```python
from build123d import *

# Parameters (mm, degrees)
BOSS_EXTRUDE1_DEPTH       = 6.35
F_6_CLEARANCE_HOLE1_D     = 3.6576
F_6_CLEARANCE_HOLE1_DEPTH = 25.4
F_6_CLEARANCE_HOLE1_TIP   = 1.0988539
FILLET1_R                 = 12.7
F_4_CLEARANCE_HOLE1_D     = 2.9464
F_4_CLEARANCE_HOLE1_DEPTH = 25.4
F_4_CLEARANCE_HOLE1_TIP   = 0.885187864
LPATTERN4_COUNT           = 6
LPATTERN4_PITCH           = 25.4
LPATTERN4_COUNT_DIR2      = 7
LPATTERN4_PITCH_DIR2      = 23.622


with BuildPart() as part:
    # Sketch1 → Boss-Extrude1 (new body)
    with BuildSketch(Plane(origin=(0, 0, 0), x_dir=(1, 0, 0), z_dir=(0, 1, 0))):
        with BuildLine():
            Line((65.058096917, 37.174573643), (142.24566953, 81.28))
            ThreePointArc((142.24566953, 81.28), (0, 163.83), (-142.24566953, 81.28))
            Line((-142.24566953, 81.28), (-65.058096917, 37.174573643))
            ThreePointArc((-65.058096917, 37.174573643), (0, 74.93), (65.058096917, 37.174573643))
        make_face()
    extrude(amount=BOSS_EXTRUDE1_DEPTH)

    # 6 Clearance Hole1
    with Locations(Plane(origin=(-50.8, 6.35, -125.73), x_dir=(0, 0, 1), z_dir=(0, 1, 0))):
        with Locations((0, 0), (0, 101.6)):
            Hole(F_6_CLEARANCE_HOLE1_D / 2, depth=F_6_CLEARANCE_HOLE1_DEPTH)
            with Locations((0, 0, -(F_6_CLEARANCE_HOLE1_DEPTH + F_6_CLEARANCE_HOLE1_TIP / 2))):  # 118° drill point
                Cone(0, F_6_CLEARANCE_HOLE1_D / 2, F_6_CLEARANCE_HOLE1_TIP, mode=Mode.SUBTRACT)

    # Fillet1
    fillet1_edges = [part.edges().sort_by_distance(p)[0] for p in [
        (142.24566953, 3.175, -81.28),
        (65.058096917, 3.175, -37.174573643),
        (-65.058096917, 3.175, -37.174573643),
        (-142.24566953, 3.175, -81.28),
    ]]
    fillet(fillet1_edges, radius=FILLET1_R)

    # 4 Clearance Hole1
    with Locations(Plane(origin=(0, 6.35, 0), x_dir=(-1, 0, 0), z_dir=(0, 1, 0))):
        with Locations((-34.0106, -133.35), (34.0106, -133.35)):
            Hole(F_4_CLEARANCE_HOLE1_D / 2, depth=F_4_CLEARANCE_HOLE1_DEPTH)
            with Locations((0, 0, -(F_4_CLEARANCE_HOLE1_DEPTH + F_4_CLEARANCE_HOLE1_TIP / 2))):  # 118° drill point
                Cone(0, F_4_CLEARANCE_HOLE1_D / 2, F_4_CLEARANCE_HOLE1_TIP, mode=Mode.SUBTRACT)

    # Sketch5 → 10 Clearance Hole1 (revolve, cut)
    with BuildSketch(Plane(origin=(-128.255094273, 6.35, -84.874017323), x_dir=(0, 0, 1), z_dir=(1, 0, 0))):
        Polygon((0, 0), (0, 26.895662253), (2.4892, 25.4), (2.4892, 0), align=None)
    f_10_clearance_hole1 = revolve(axis=Axis((-128.255094273, 12.7, -84.874017323), (0, -1, 0)), mode=Mode.SUBTRACT)

    # LPattern4: 10 Clearance Hole1 6 × 7, 28 skipped
    with Locations(*[Vector(0, 0, -1) * (i * LPATTERN4_PITCH) + Vector(0.8667949394357126, 0, 0.49866475007628064) * (j * LPATTERN4_PITCH_DIR2) for i in range(LPATTERN4_COUNT) for j in range(LPATTERN4_COUNT_DIR2) if (i, j) not in ((0, 0), (0, 4), (0, 5), (0, 6), (1, 0), (1, 4), (1, 5), (1, 6), (2, 0), (2, 1), (2, 4), (2, 6), (3, 0), (3, 1), (3, 2), (3, 4), (3, 6), (4, 0), (4, 1), (4, 2), (4, 3), (4, 4), (4, 6), (5, 0), (5, 1), (5, 2), (5, 3), (5, 4), (5, 6))]):
        add(f_10_clearance_hole1, mode=Mode.SUBTRACT)

    # Mirror4: 10 Clearance Hole1 across plane
    add(f_10_clearance_hole1.mirror(Plane(origin=(0, 0, 0), x_dir=(0, 0, 1), z_dir=(1, 0, 0))), mode=Mode.SUBTRACT)

    # Mirror4 copy 1 sketch → Mirror4 copy 1 (revolve, cut)
    with BuildSketch(Plane(origin=(107.779664214, 6.35, -73.094558596), x_dir=(0, 0, 1), z_dir=(-1, 0, 0))):
        Polygon((0, 0), (0, -26.895662253), (2.4892, -25.4), (2.4892, 0), align=None)
    revolve(axis=Axis((107.779664214, 12.7, -73.094558596), (0, 1, 0)), mode=Mode.SUBTRACT)

    # Mirror4 copy 2 sketch → Mirror4 copy 2 (revolve, cut)
    with BuildSketch(Plane(origin=(87.304234155, 6.35, -61.31509987), x_dir=(0, 0, 1), z_dir=(-1, 0, 0))):
        Polygon((0, 0), (0, -26.895662253), (2.4892, -25.4), (2.4892, 0), align=None)
    revolve(axis=Axis((87.304234155, 12.7, -61.31509987), (0, 1, 0)), mode=Mode.SUBTRACT)

    # Mirror4 copy 3 sketch → Mirror4 copy 3 (revolve, cut)
    with BuildSketch(Plane(origin=(66.828804095, 6.35, -49.535641144), x_dir=(0, 0, 1), z_dir=(-1, 0, 0))):
        Polygon((0, 0), (0, -26.895662253), (2.4892, -25.4), (2.4892, 0), align=None)
    revolve(axis=Axis((66.828804095, 12.7, -49.535641144), (0, 1, 0)), mode=Mode.SUBTRACT)

    # Mirror4 copy 4 sketch → Mirror4 copy 4 (revolve, cut)
    with BuildSketch(Plane(origin=(107.779664214, 6.35, -98.494558596), x_dir=(0, 0, 1), z_dir=(-1, 0, 0))):
        Polygon((0, 0), (0, -26.895662253), (2.4892, -25.4), (2.4892, 0), align=None)
    revolve(axis=Axis((107.779664214, 12.7, -98.494558596), (0, 1, 0)), mode=Mode.SUBTRACT)

    # Mirror4 copy 5 sketch → Mirror4 copy 5 (revolve, cut)
    with BuildSketch(Plane(origin=(87.304234155, 6.35, -86.71509987), x_dir=(0, 0, 1), z_dir=(-1, 0, 0))):
        Polygon((0, 0), (0, -26.895662253), (2.4892, -25.4), (2.4892, 0), align=None)
    revolve(axis=Axis((87.304234155, 12.7, -86.71509987), (0, 1, 0)), mode=Mode.SUBTRACT)

    # Mirror4 copy 6 sketch → Mirror4 copy 6 (revolve, cut)
    with BuildSketch(Plane(origin=(66.828804095, 6.35, -74.935641144), x_dir=(0, 0, 1), z_dir=(-1, 0, 0))):
        Polygon((0, 0), (0, -26.895662253), (2.4892, -25.4), (2.4892, 0), align=None)
    revolve(axis=Axis((66.828804095, 12.7, -74.935641144), (0, 1, 0)), mode=Mode.SUBTRACT)

    # Mirror4 copy 7 sketch → Mirror4 copy 7 (revolve, cut)
    with BuildSketch(Plane(origin=(87.304234155, 6.35, -112.11509987), x_dir=(0, 0, 1), z_dir=(-1, 0, 0))):
        Polygon((0, 0), (0, -26.895662253), (2.4892, -25.4), (2.4892, 0), align=None)
    revolve(axis=Axis((87.304234155, 12.7, -112.11509987), (0, 1, 0)), mode=Mode.SUBTRACT)

    # Mirror4 copy 8 sketch → Mirror4 copy 8 (revolve, cut)
    with BuildSketch(Plane(origin=(66.828804095, 6.35, -100.335641144), x_dir=(0, 0, 1), z_dir=(-1, 0, 0))):
        Polygon((0, 0), (0, -26.895662253), (2.4892, -25.4), (2.4892, 0), align=None)
    revolve(axis=Axis((66.828804095, 12.7, -100.335641144), (0, 1, 0)), mode=Mode.SUBTRACT)

    # Mirror4 copy 9 sketch → Mirror4 copy 9 (revolve, cut)
    with BuildSketch(Plane(origin=(25.877943977, 6.35, -76.776723691), x_dir=(0, 0, 1), z_dir=(-1, 0, 0))):
        Polygon((0, 0), (0, -26.895662253), (2.4892, -25.4), (2.4892, 0), align=None)
    revolve(axis=Axis((25.877943977, 12.7, -76.776723691), (0, 1, 0)), mode=Mode.SUBTRACT)

    # Mirror4 copy 10 sketch → Mirror4 copy 10 (revolve, cut)
    with BuildSketch(Plane(origin=(66.828804095, 6.35, -125.735641144), x_dir=(0, 0, 1), z_dir=(-1, 0, 0))):
        Polygon((0, 0), (0, -26.895662253), (2.4892, -25.4), (2.4892, 0), align=None)
    revolve(axis=Axis((66.828804095, 12.7, -125.735641144), (0, 1, 0)), mode=Mode.SUBTRACT)

    # Mirror4 copy 11 sketch → Mirror4 copy 11 (revolve, cut)
    with BuildSketch(Plane(origin=(25.877943977, 6.35, -102.176723691), x_dir=(0, 0, 1), z_dir=(-1, 0, 0))):
        Polygon((0, 0), (0, -26.895662253), (2.4892, -25.4), (2.4892, 0), align=None)
    revolve(axis=Axis((25.877943977, 12.7, -102.176723691), (0, 1, 0)), mode=Mode.SUBTRACT)

    # Mirror4 copy 12 sketch → Mirror4 copy 12 (revolve, cut)
    with BuildSketch(Plane(origin=(25.877943977, 6.35, -127.576723691), x_dir=(0, 0, 1), z_dir=(-1, 0, 0))):
        Polygon((0, 0), (0, -26.895662253), (2.4892, -25.4), (2.4892, 0), align=None)
    revolve(axis=Axis((25.877943977, 12.7, -127.576723691), (0, 1, 0)), mode=Mode.SUBTRACT)

    # Mirror4 copy 13 sketch → Mirror4 copy 13 (revolve, cut)
    with BuildSketch(Plane(origin=(25.877943977, 6.35, -152.976723691), x_dir=(0, 0, 1), z_dir=(-1, 0, 0))):
        Polygon((0, 0), (0, -26.895662253), (2.4892, -25.4), (2.4892, 0), align=None)
    revolve(axis=Axis((25.877943977, 12.7, -152.976723691), (0, 1, 0)), mode=Mode.SUBTRACT)


solid = part.part
```
Here's how the part is built. I have some questions about the finished solid (model axes, mm). Round coordinates to 2 decimals unless told otherwise and drop trailing zeros. Write each loop counter-clockwise with the first axis right and the second up, starting at its lowest first coordinate (ties: lowest second). Pieces come first, ordered by that corner, then holes.
Q1. Please list where these lines run through material, in increasing order: probe 1 along X at (y, z) = (1, -49); probe 2 along X at (y, z) = (5.5, -85.5); probe 3 along X at (y, z) = (3.25, -129).
Q2. If we section it at A-A on y = 4.25: Give the number of separate pieces and of enclosed holes in the cut face, plus the area to 3 significant figures.
Q3. If we section it at B-B on x = -13: Write out the boundary of the cut face in (y, z), plus the area to 3 significant figures.
Q4. If we mould it in two halves opening along Z, with no side actions, what happens to faces 1 (the cylindrical face through (2.219, 3.131, -163.815)), 2 (the cylindrical face through (87.414, 3.219, -63.802)), 3 (the flat face through (-2, 6.35, -103)), 4 (the flat face through (102.63, 3.131, -58.643))? For each: +Z half, -Z half, draft (parallel to the pull), parting line (faces both ways), or undercut.
Q5. Will these pins go through, and if not, where does the flat tip stop? P1, Ø2, axis at x = 50.5, y = 4, coming from the +Z side; P2, Ø1.5, axis at x = 32, y = 3.5, coming from the -Z side.
Answer below:
1. probe 1: x = -85.75 to -69.26, -64.4 to -56.69, 56.69 to 64.4, 69.26 to 85.75
1. probe 2: x = -137.15 to -130.66, -125.85 to -89.48, -85.13 to 85.13, 89.48 to 125.85, 130.66 to 137.15
1. probe 3: x = -100.99 to -27.92, -23.84 to 23.84, 27.92 to 100.99
2. separate pieces: 1
2. enclosed holes: 32
2. area: 21,600 mm2
3. outline: (0, -163.31) - (6.35, -163.31) - (6.35, -73.79) - (0, -73.79) - close
3. area: 568 mm2
4. face 1: -Z half
4. face 2: undercut
4. face 3: draft
4. face 4: +Z half
5. P1: stops at z = -54.43
5. P2: stops at z = -160.82
